```python
from build123d import *

# Parameters (mm, degrees)
SKETCH1_W           = 4
SKETCH1_H           = 15
BOSS_EXTRUDE1_DEPTH = 4


with BuildPart() as part:
    # Sketch1 → Boss-Extrude1 (new body)
    with BuildSketch(Plane.XY):
        Polygon((-75, -50), (75, -50), (110, -50), (110, 50), (75, 50), (-75, 50), align=None)
        with Locations((58, 27.5)):
            Rectangle(SKETCH1_W, SKETCH1_H, mode=Mode.SUBTRACT)
        with Locations((58, -27.5)):
            Rectangle(SKETCH1_W, SKETCH1_H, mode=Mode.SUBTRACT)
        with Locations((-58, 27.5)):
            Rectangle(SKETCH1_W, SKETCH1_H, mode=Mode.SUBTRACT)
        with Locations((-58, -27.5)):
            Rectangle(SKETCH1_W, SKETCH1_H, mode=Mode.SUBTRACT)
        with Locations((103, 27.5)):
            Rectangle(SKETCH1_W, SKETCH1_H, mode=Mode.SUBTRACT)
        with Locations((103, -27.5)):
            Rectangle(SKETCH1_W, SKETCH1_H, mode=Mode.SUBTRACT)
    extrude(amount=BOSS_EXTRUDE1_DEPTH)


solid = part.part
```
The model under review builds one solid part; all positions refer to its coordinate system, in mm. A direction names the side the tool comes from. Coordinates: 2 decimals unless noted, no trailing zeros. Write each loop counter-clockwise with the first axis right and the second up, starting at its lowest first coordinate (ties: lowest second). Pieces come first, ordered by that corner, then holes. Notation, with made-up numbers: (-10, -14) - (4, -14) arc R5 ccw to (4, -7) - close; hole circle Ø6 at (23, 69.25). An arc over 180 degrees is marked (long way). Write item = value, one per line.
(1) Consider section B-B, the plane y = -28.5. Give the boundary of the cut face in (x, z), then the cut area to 3 significant figures.
Result sheet:
outline = (-75, 0) - (-60, 0) - (-60, 4) - (-75, 4) - close; (-56, 0) - (56, 0) - (56, 4) - (-56, 4) - close; (60, 0) - (101, 0) - (101, 4) - (60, 4) - close; (105, 0) - (110, 0) - (110, 4) - (105, 4) - close
area = 692 mm^2
(2) For P1, Ø1, axis at x = 30.5, y = 7.5, coming from the -Z side, flat-tipped, find the tip position at first contact; note if it passes through.
Result sheet:
P1 = 0
(3) Mouldability with a two-part tool opening along X and no side actions: class faces 1 (the face through (110, -1, 2)), 2 (the face through (19, 50, 2)), 3 (the face through (-58, -35, 2)) as pulls with the +X half, pulls with the -X half, needs draft (parallel to the pull), parting line crosses it, or undercut.
Result sheet:
face_1 = pulls with the +X half
face_2 = needs draft
face_3 = undercut
(4) Consider section A-A, the plane z = 1.5. Give the boundary of the cut face in (x, y).
Result sheet:
outline = (-75, -50) - (110, -50) - (110, 50) - (-75, 50) - close; hole (-60, -35) - (-56, -35) - (-56, -20) - (-60, -20) - close; hole (-60, 20) - (-56, 20) - (-56, 35) - (-60, 35) - close; hole (56, -35) - (60, -35) - (60, -20) - (56, -20) - close; hole (56, 20) - (60, 20) - (60, 35) - (56, 35) - close; hole (101, -35) - (105, -35) - (105, -20) - (101, -20) - close; hole (101, 20) - (105, 20) - (105, 35) - (101, 35) - close
(5) Machinability: for faces 4 (the face through (16, -50, 2)), 5 (the face through (56, 27, 2)), which of the approach directions +Z, -Z, +X, -X, +Y, -Y give a long, thin tool a straight path to every point of the face, cutting with its end or side? Answer none if there is none.
Result sheet:
face_4 = +Z, -Z, +X, -X, -Y
face_5 = +Z, -Z
(6) For line 1 (X direction, y = -30, z = 3), list the stretches that pass through material, from the lowest coordinate up. Write a range as [from, to].
Result sheet:
line_1 = [-75, -60], [-56, 56], [60, 101], [105, 110]
